```python
from build123d import *

# Parameters (mm, degrees)
SKETCH_1_R      = 2
SKETCH_1_W      = 42.5
SKETCH_1_H      = 62.5
SKETCH_1_W_2    = 6
EXTRUDE_1_DEPTH = 5


with BuildPart() as part:
    # 草图1 → 凸台-拉伸1 (new body)
    with BuildSketch(Plane.XY):
        Polygon((1909.377089995, 1448.678588443), (2093.877089995, 1448.678588443), (2093.877089995, 1455.029082267), (2087.877089995, 1455.029082267), (2087.877089995, 1517.529082267), (2093.877089995, 1517.529082267), (2093.877089995, 1523.678588443), (1909.377089995, 1523.678588443), (1909.377089995, 1517.529082267), (1915.377089995, 1517.529082267), (1915.377089995, 1455.029082267), (1909.377089995, 1455.029082267), align=None)
        with Locations((1918.127089995, 1453.029082267)):
            Circle(SKETCH_1_R, mode=Mode.SUBTRACT)
        with Locations((1966.127089995, 1453.029082267)):
            Circle(SKETCH_1_R, mode=Mode.SUBTRACT)
        with Locations((1977.627089995, 1453.029082267)):
            Circle(SKETCH_1_R, mode=Mode.SUBTRACT)
        with Locations((2025.627089995, 1453.029082267)):
            Circle(SKETCH_1_R, mode=Mode.SUBTRACT)
        with Locations((2037.127089995, 1453.029082267)):
            Circle(SKETCH_1_R, mode=Mode.SUBTRACT)
        with Locations((2085.127089995, 1453.029082267)):
            Circle(SKETCH_1_R, mode=Mode.SUBTRACT)
        with Locations((1942.127089995, 1486.279082267)):
            Rectangle(SKETCH_1_W, SKETCH_1_H, mode=Mode.SUBTRACT)
        Polygon((1968.877089995, 1455.029082267), (1968.877089995, 1486.279082267), (1968.877089995, 1517.529082267), (1974.877089995, 1517.529082267), (1974.877089995, 1455.029082267), align=None, mode=Mode.SUBTRACT)
        with Locations((1918.127089995, 1519.529082267)):
            Circle(SKETCH_1_R, mode=Mode.SUBTRACT)
        with Locations((1966.127089995, 1519.529082267)):
            Circle(SKETCH_1_R, mode=Mode.SUBTRACT)
        with Locations((1977.627089995, 1519.529082267)):
            Circle(SKETCH_1_R, mode=Mode.SUBTRACT)
        with Locations((2001.627089995, 1486.279082267)):
            Rectangle(SKETCH_1_W, SKETCH_1_H, mode=Mode.SUBTRACT)
        with Locations((2031.377089995, 1486.279082267)):
            Rectangle(SKETCH_1_W_2, SKETCH_1_H, mode=Mode.SUBTRACT)
        with Locations((2061.127089995, 1486.279082267)):
            Rectangle(SKETCH_1_W, SKETCH_1_H, mode=Mode.SUBTRACT)
        with Locations((2025.627089995, 1519.529082267)):
            Circle(SKETCH_1_R, mode=Mode.SUBTRACT)
        with Locations((2037.127089995, 1519.529082267)):
            Circle(SKETCH_1_R, mode=Mode.SUBTRACT)
        with Locations((2085.127089995, 1519.529082267)):
            Circle(SKETCH_1_R, mode=Mode.SUBTRACT)
    extrude(amount=EXTRUDE_1_DEPTH)


solid = part.part
```
Check sheet for the modelled part. Datum: model origin and axes. Units: mm. A direction names the side the tool comes from. Coordinates: 2 decimals unless noted, no trailing zeros. Order: outer loops, then holes, each group sorted by start corner. A loop starts at its lowest first (then second) coordinate and runs counter-clockwise, first axis right, second up. Notation, with made-up numbers: M -4,56.5 L 38,56.5 A18 ccw 38,86.5 Z; hole C -6,71 d9. An arc over 180 degrees is marked long. One line per question, with ' | ' between items. Start each with the question number.
Item 1: Sectioned sample at B-B on y = 1473.5. Record the cut outline in (x, z), and give its area (3 significant figures).
Item 2: Sectioned sample at A-A on x = 2050. Record the cut outline in (y, z).
Item 3: Gauge pin test, flat ends, axial feed: P1, Ø2.5, axis at y = 1475.5, z = 2.5, coming from the -X side; P2, Ø3, axis at x = 2037.13, y = 1453.03, coming from the -Z side; P3, Ø1.5, axis at y = 1484, z = 2, coming from the +X side; P4, Ø5, axis at x = 2085.13, y = 1453.03, coming from the +Z side. Record the tip position at first contact, or that the pin passes through.
Item 4: Access from +Z, -Z, +X, -X, +Y, -Y to the whole of each face (thin tool, end or side, straight path). Record for faces 1 (the flat face through (2061, 1517.529, 2)), 2 (the flat face through (2087.877, 1486, 2)), 3 (the flat face through (1980, 1487, 5)).
Item 5: Mould release check, pull along X, two halves, no side actions. Record for faces 4 (the flat face through (2031, 1517.529, 2)), 5 (the flat face through (2091, 1455.029, 2)), 6 (the flat face through (2093.877, 1452, 2)): pulls with the +X half, pulls with the -X half, needs draft (parallel to the pull), parting line crosses it, or undercut.
Item 6: Material ranges on line 1 (Y direction, x = 2025.5, z = 1.5); line 2 (X direction, y = 1512.5, z = 4.25); line 3 (Y direction, x = 1930.5, z = 2), recorded low to high.
Item 7: Sectioned sample at C-C on z = 4.25. Count the separate pieces of the cut face and the enclosed holes in it, and give its area (3 significant figures).
Answer below:
1) outline: M 1915.38,0 L 1920.88,0 L 1920.88,5 L 1915.38,5 Z; M 1963.38,0 L 1968.88,0 L 1968.88,5 L 1963.38,5 Z; M 1974.88,0 L 1980.38,0 L 1980.38,5 L 1974.88,5 Z; M 2022.88,0 L 2028.38,0 L 2028.38,5 L 2022.88,5 Z; M 2034.38,0 L 2039.88,0 L 2039.88,5 L 2034.38,5 Z; M 2082.38,0 L 2087.88,0 L 2087.88,5 L 2082.38,5 Z | area: 165 mm^2
2) outline: M 1448.68,0 L 1455.03,0 L 1455.03,5 L 1448.68,5 Z; M 1517.53,0 L 1523.68,0 L 1523.68,5 L 1517.53,5 Z
3) P1: stops at x = 1915.38 | P2: passes through | P3: stops at x = 2087.88 | P4: stops at z = 5
4) face 1: +Z, -Z | face 2: +Z, -Z, +X | face 3: +Z, +X, -X, +Y, -Y
5) face 4: undercut | face 5: needs draft | face 6: pulls with the +X half
6) line 1: y = 1448.68 to 1451.03, 1455.03 to 1517.53, 1521.53 to 1523.68 | line 2: x = 1915.38 to 1920.88, 1963.38 to 1968.88, 1974.88 to 1980.38, 2022.88 to 2028.38, 2034.38 to 2039.88, 2082.38 to 2087.88 | line 3: y = 1448.68 to 1455.03, 1517.53 to 1523.68
7) separate pieces: 1 | enclosed holes: 17 | area: 4,220 mm^2
